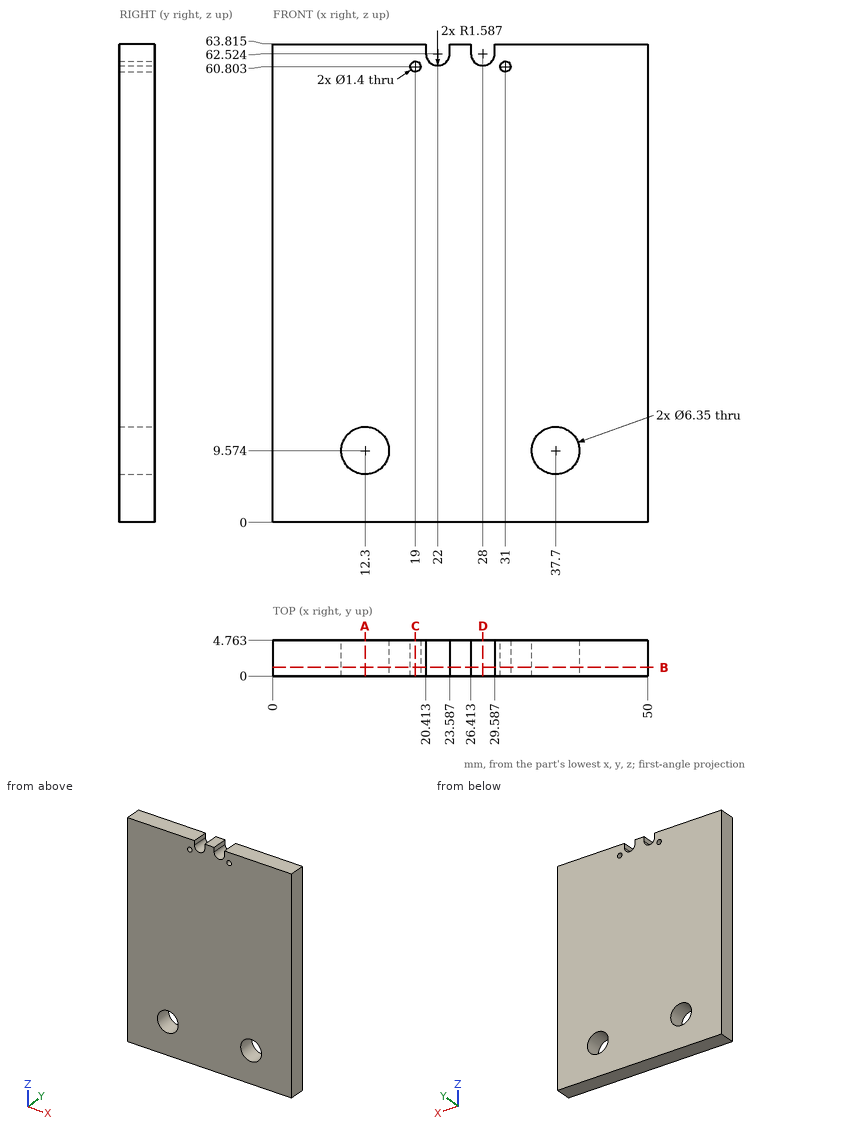
Source: three-view drawing plus pictorial views. Frame: mm from the lowest corner of the part. Give positions to 0.01 mm unless a question says otherwise; leave off trailing zeros. Loops run counter-clockwise (first coordinate to the right, second up) from the corner with the lowest first, then second, coordinate; pieces in that order, holes last. Notation, with made-up numbers: (7.25, 9) -> (58.25, 9) arc R27 ccw to (58.25, 41) -> close; hole circle Ø1 at (-26.75, 18). An arc over 180 degrees is marked (long way). Use a Markdown table: item, result. Add a question column.
(1) Section query D-D (x = 28). Output: boundary loops of the cut face in (y, z).
(2) Section query B-B (y = 1.15). Count the separate pieces of the cut face and the enclosed holes in it, then the cut area to 3 significant figures.
(3) Section query C-C (x = 19). Output: boundary loops of the cut face in (y, z) (1 decimal), then the cut area to 3 significant figures.
(4) First-contact query: pin 1 Ø5.5 at (x, z) = (37.7, 9.57) entering from +Y; pin 2 Ø1.5 at (y, z) = (2, 47.5) entering from -X. Flat tips, straight axial feed; report the tip coordinate or a pass-through.
(5) Section query A-A (x = 12.3). Output: boundary loops of the cut face in (y, z) (1 decimal), then the cut area to 3 significant figures.
(6) Ray query, line 1 (Z direction, x = 37.7, y = 3.7) (1 decimal); line 2 (Z direction, x = 19, y = 1.85) (1 decimal); line 3 (X direction, y = 4.1, z = 10.5). Return the intervals inside material, ascending.
Checked values:
| question | item | result |
|---|---|---|
| 1 | outline | (0, 0) -> (4.76, 0) -> (4.76, 60.94) -> (0, 60.94) -> close |
| 2 | separate pieces | 1 |
| 2 | enclosed holes | 4 |
| 2 | area | 3,110 mm^2 |
| 3 | outline | (0, 0) -> (4.8, 0) -> (4.8, 60.1) -> (0, 60.1) -> close; (0, 61.5) -> (4.8, 61.5) -> (4.8, 63.8) -> (0, 63.8) -> close |
| 3 | area | 297 mm^2 |
| 4 | pin 1 | through |
| 4 | pin 2 | x = 0 |
| 5 | outline | (0, 0) -> (4.8, 0) -> (4.8, 6.4) -> (0, 6.4) -> close; (0, 12.7) -> (4.8, 12.7) -> (4.8, 63.8) -> (0, 63.8) -> close |
| 5 | area | 274 mm^2 |
| 6 | line 1 | 0 to 6.4, 12.7 to 63.8 |
| 6 | line 2 | 0 to 60.1, 61.5 to 63.8 |
| 6 | line 3 | 0 to 9.26, 15.34 to 34.66, 40.74 to 50 |
